Verification items for the finished model (mm, model axes). A direction names the side the tool comes from. Coordinates: 2 decimals unless noted, no trailing zeros. Write each loop counter-clockwise with the first axis right and the second up, starting at its lowest first coordinate (ties: lowest second). Pieces come first, ordered by that corner, then holes. Notation, with made-up numbers: (5.5, 20) -> (47.5, 20) arc R20 cw to (47.5, 56) -> close; hole circle Ø11 at (37.5, 24.5). An arc over 180 degrees is marked (long way). Use a Markdown table: item, result. Add a question column.
Solid Edge part; units mm, degrees
sketch "Sketch1" plane through (0, 0, 0) normal (0, 0, 1) x (1, 0, 0)
  circle A0 centre (0, 0) radius 3
extrude "Protrusion1" add sketch "Sketch1" along normal blind 1.7
sketch "Sketch2" plane through (0, 0, 0) normal (0, 0, -1) x (1, 0, 0)
  circle A0 centre (0, 0) radius 1.5
extrude "Protrusion2" add sketch "Sketch2" along normal blind 10.3
sketch "Sketch3" plane through (0, 0, -10.3) normal (0, 0, -1) x (1, 0, 0)
  circle A0 centre (0, 0) radius 1.4997
extrude "Cutout1" cut sketch "Sketch3" against normal blind 10.2897 flip side to cut
chamfer "Chamfer_1" distance 0.225 angle 45 1 edges at (-1.4997, 0, -10.3)
sketch "Sketch4" plane through (0, 0, 1.7) normal (0, 0, 1) x (1, 0, 0)
  line L0 (-0.5774, 1) -> (0.5774, 1)
  line L1 (1.1547, 0) -> (0.5774, 1)
  line L2 (0.5774, -1) -> (1.1547, 0)
  line L3 (-0.5774, -1) -> (0.5774, -1)
  line L4 (-1.1547, 0) -> (-0.5774, -1)
  line L5 (-0.5774, 1) -> (-1.1547, 0)
extrude "Cutout2" cut sketch "Sketch4" against normal blind 1.1333
sketch "Sketch5" plane through (0, 0, 0) normal (0, -1, 0) x (1, 0, 0)
  line L0 (3, 1.7) -> (1.3, 0)
  line L1 (1.3, 0) -> (3, 0)
  line L2 (3, 0) -> (3, 1.7)
revolve "RevolvedCutout1" cut sketch "Sketch5" angle 360 about axis through (0, 0, 14.0017) along (0, 0, -1)
properties part number "133795"
1) Cross-section at B-B on z = -7.75. Record the boundary of the cut face in (x, y), then the cut area to 3 significant figures.
2) Set-up check for faces 1 (the face through (0, -1.3, 1.7)), 2 (the face through (0.87, 0.49, 1.14)): record each of +Z, -Z, +X, -X, +Y, -Y from which the full face is reachable in a straight line by a thin tool's end or side.
3) Gauge pin test, flat ends, axial feed: pin 1 (1.5 mm diameter, centred on x = -0.5, z = -1, fed in from +Y); pin 2 (1.5 mm diameter, centred on x = -1, z = -2, fed in from -Y); pin 3 (3 mm diameter, centred on x = 2, y = -2, fed in from -Z). Record the tip position at first contact, or that the pin passes through.
4) Thickness scan on L1, parallel to X at y = -1.3, z = -9.5; L2, parallel to Z at x = -1.75, y = -0.2; L3, parallel to Y at x = 1.1, z = -3.25. Record the ranges inside material, lowest first.
5) Release check for a two-part mould opening along Y. For faces 3 (the face through (-0.325, 1.464, -5.113)), 4 (the face through (0, 0, -10.3)), 5 (the face through (0.86, -0.51, 1.14)) record: released by +Y, released by -Y, zero draft, split by the parting line, or undercut.
Returned:
| question | item | result |
|---|---|---|
| 1 | outline | circle Ø3 at (0, 0) |
| 1 | area | 7.07 mm² |
| 2 | face 1 | +Z, +X, -X, +Y, -Y |
| 2 | face 2 | +Z |
| 3 | pin 1 | stops at y = 1.5 |
| 3 | pin 2 | stops at y = -1.48 |
| 3 | pin 3 | stops at z = -10.25 |
| 4 | L1 | x = -0.75 to 0.75 |
| 4 | L2 | z = 0.46 to 1.7 |
| 4 | L3 | y = -1.02 to 1.02 |
| 5 | face 3 | split by the parting line |
| 5 | face 4 | zero draft |
| 5 | face 5 | undercut |
